Source: three-view drawing plus pictorial views. Frame: mm from the lowest corner of the part. A direction names the side the tool comes from. Give positions to 0.01 mm unless a question says otherwise; leave off trailing zeros. Order: outer loops, then holes, each group sorted by start corner. A loop starts at its lowest first (then second) coordinate and runs counter-clockwise, first axis right, second up. Notation, with made-up numbers: (24.25, 10.5) -> (43.25, 10.5) arc R8 ccw to (43.25, 15.5) -> close; hole circle Ø4 at (10.5, 40). An arc over 180 degrees is marked (long way). Answer in a Markdown table with one row per item.
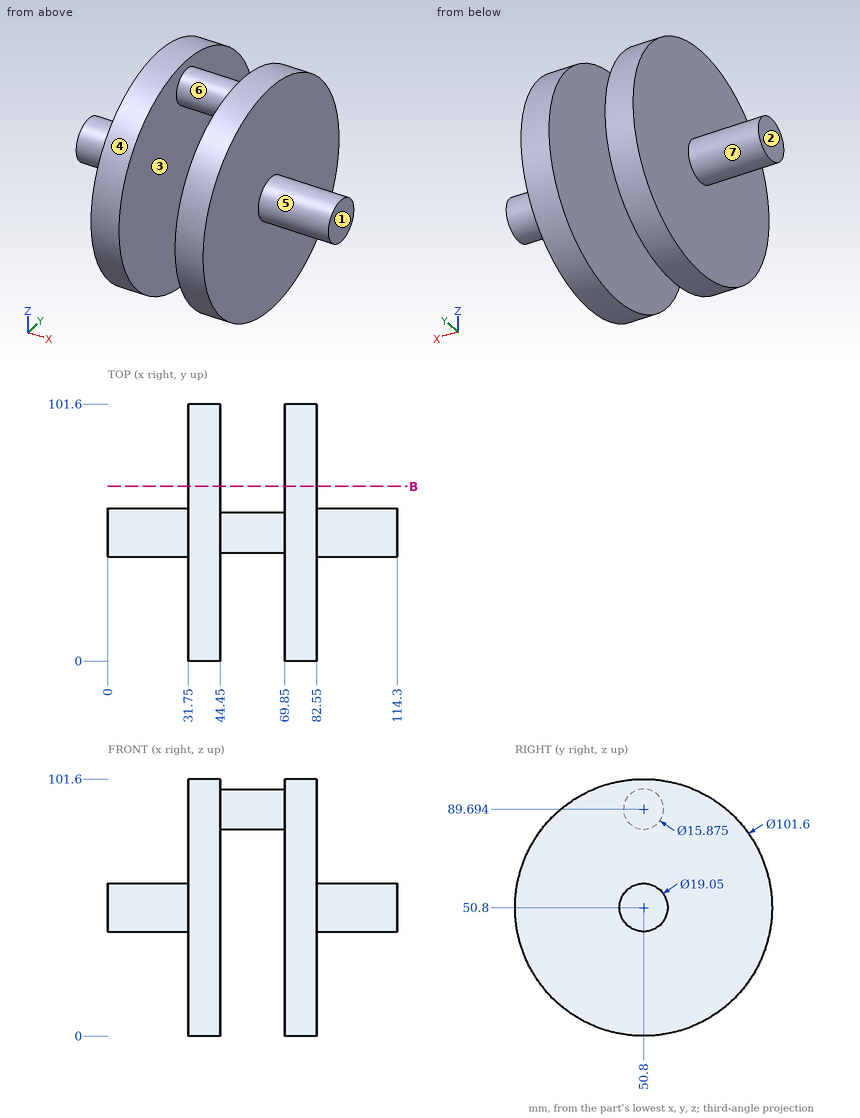
(1) Access query for the marked faces 4, 5, 6 and 7. Directions: +Z, -Z, +X, -X, +Y, -Y. A direction counts if a zero-diameter tool reaches every point of the face in a straight line with its end or side. Return the directions, or none.
A:
| item | result |
|---|---|
| face 4 | +X, -X |
| face 5 | +X |
| face 6 | none |
| face 7 | -X |
(2) Ray query, probe 1 along X at (y, z) = (54, 5.5); probe 2 along Z at (x, y) = (36.5, 64) (1 decimal); probe 3 along Y at (x, z) = (82.5, 17.5). Return the intervals inside material, ascending.
A:
| item | result |
|---|---|
| probe 1 | x = 31.75 to 44.45, 69.85 to 82.55 |
| probe 2 | z = 1.7 to 99.9 |
| probe 3 | y = 12.44 to 89.16 |
(3) First-contact query: pin 1 Ø8 at (y, z) = (41.5, 81.5) entering from +X; pin 2 Ø10 at (x, z) = (99, 63) entering from +Y (1 decimal); pin 3 Ø10 at (x, y) = (64, 54) entering from +Z. Flat tips, straight axial feed; report the tip coordinate or a pass-through.
A:
| item | result |
|---|---|
| pin 1 | stops at x = 82.55 |
| pin 2 | stops at y = 57 |
| pin 3 | stops at z = 97.63 |
(4) Pull-direction query (X, two-part tool) for the marked faces 1, 2 and 3; classes: +X half, -X half, draft (parallel to the pull), parting line (faces both ways), or undercut.
A:
| item | result |
|---|---|
| face 1 | +X half |
| face 2 | -X half |
| face 3 | undercut |
(5) Section query B-B (y = 69). Return the cut outline in (x, z).
A:
| item | result |
|---|---|
| outline | (31.75, 3.37) -> (44.45, 3.37) -> (44.45, 98.23) -> (31.75, 98.23) -> close; (69.85, 3.37) -> (82.55, 3.37) -> (82.55, 98.23) -> (69.85, 98.23) -> close |
